Verification items for the finished model (mm, model axes). Round coordinates to 2 decimals unless told otherwise and drop trailing zeros. Write each loop counter-clockwise with the first axis right and the second up, starting at its lowest first coordinate (ties: lowest second). Pieces come first, ordered by that corner, then holes. Notation, with made-up numbers: M 89,60 L 108,60 A23 cw 108,75 Z; hole C -10,29.25 d5. An arc over 180 degrees is marked long. Use a Markdown table: item, result. Add a question column.
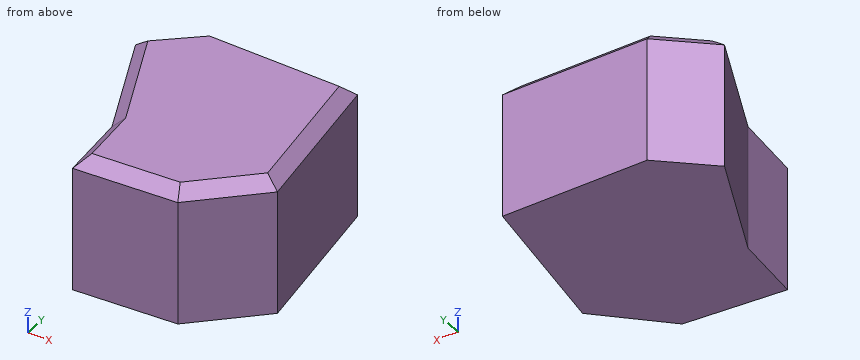
from build123d import *

# Parameters (mm, degrees)
F1_DEPTH = 58.443097
F2_SIZE  = 5.08


with BuildPart() as f1:
    # F0 (on Top) → F1 (new body)
    with BuildSketch(Plane.XY):
        with BuildLine():
            Line((-18.330865, 29.696003), (-39.228059, 11.548445))
            add(Edge.make_bspline(
                [(-19.247405, -34.095421), (-25.907624, -18.880798), (-32.567841, -3.666179), (-39.228059, 11.548445)],
                knots=[0, 0, 0, 0, 49.825586, 49.825586, 49.825586, 49.825586], degree=3))
            Line((-19.247405, -34.095421), (-17.23101, -62.691584))
            Line((-17.23101, -62.691584), (25.296614, -59.392035))
            Line((25.296614, -59.392035), (51.326454, -34.645349))
            Line((51.326454, -34.645349), (43.077558, 29.696003))
            Line((43.077558, 29.696003), (-18.330865, 29.696003))
        make_face()
    extrude(amount=F1_DEPTH)

    # F2
    f2_edges = [f1.edges().sort_by_distance(p)[0] for p in [
        (38.311534, -47.018692, 58.443097),
        (47.202006, -2.474673, 58.443097),
        (12.373347, 29.696003, 58.443097),
        (-28.779462, 20.622224, 58.443097),
        (-29.237732, -11.273488, 58.443097),
        (-18.239208, -48.393503, 58.443097),
        (4.032802, -61.04181, 58.443097),
    ]]
    chamfer(f2_edges, length=F2_SIZE)


solid = f1.part
1. Scan lines: line 1 along Z through (x, y) = (37.5, -46); line 2 along X through (y, z) = (-1.5, 53); line 3 along X through (y, z) = (-32, 48). Record each from-to range of solid material in increasing order. Write a range as from..to.
2. Depth check by flat-ended pin: pin 1 Ø2 at (y, z) = (19, 51) entering from +X; pin 2 Ø1 at (x, z) = (-4, 35.5) entering from -Y; pin 3 Ø10 at (y, z) = (6.5, 28) entering from -X. Enter the tip coordinate at first touch or a pass-through.
3. Cross-section at B-B on y = -51.5. Enter the section's corners in (x, z).
4. Cross-section at A-A on x = 33. Enter the section's corners in (y, z).
Answer:
| question | item | result |
|---|---|---|
| 1 | line 1 | z = 0..54.66 |
| 1 | line 2 | x = -33.52..47.08 |
| 1 | line 3 | x = -20.16..50.99 |
| 2 | pin 1 | stops at x = 44.58 |
| 2 | pin 2 | stops at y = -61.7 |
| 2 | pin 3 | stops at x = -39.21 |
| 3 | outline | M -18.02,0 L 33.6,0 L 33.6,53.36 L 26.23,58.44 L -12.93,58.44 L -18.02,53.36 Z |
| 4 | outline | M -52.07,0 L 29.7,0 L 29.7,53.36 L 24.62,58.44 L -45.06,58.44 L -52.07,53.36 Z |
